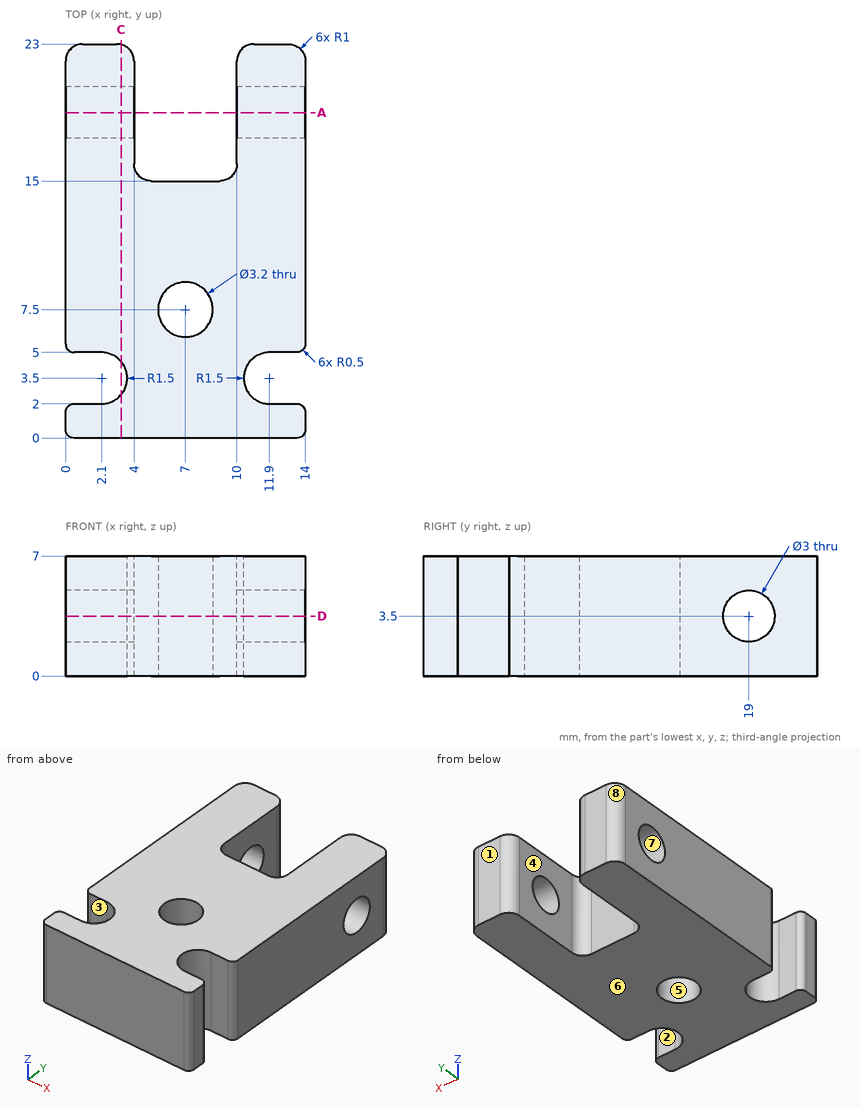
For this review, use the dimensioned drawing (mm, ordinates from the lowest corner) and the shaded views. A direction names the side the tool comes from. Coordinates: 2 decimals unless noted, no trailing zeros. Loops run counter-clockwise (first coordinate to the right, second up) from the corner with the lowest first, then second, coordinate; pieces in that order, holes last. Notation, with made-up numbers: (82, 61.5) - (135, 61.5) arc R16 ccw to (135, 91.5) - close; hole circle Ø5 at (28, 23). An arc over 180 degrees is marked (long way). Use CSV: the item, a comma, the result in double quotes. Start each with the question number.
1) Consider section D-D on z = 3.5. Give the number of separate pieces and of enclosed holes in the cut face, then the cut area to 3 significant figures.
2) Consider section A-A on y = 19. Write out the cut boundary in (x, z).
3) Tool access review of the marked faces 1, 2, 3, 4 and 5: name each direction out of +Z, -Z, +X, -X, +Y, -Y from which nothing blocks a thin tool from reaching the whole face with its end or side.
4) Consider section C-C on x = 3.25. Write out the cut boundary in (y, z), then the cut area to 3 significant figures.
5) The part is to be moulded in two halves that separate along Z. For the marked faces 6, 7 and 8, say which applies: +Z half, -Z half, draft (parallel to the pull), parting line (faces both ways), or undercut.
6) For pin 1 Ø3 at (y, z) = (19, 3) entering from +X; pin 2 Ø1.5 at (x, z) = (4.5, 5) entering from +Y, all flat-tipped, find the tip position at first contact; note any pin that passes through.
7) Wall thickness on L1, parallel to Y at x = 1.1, z = 3.5; L2, parallel to Y at x = 12.5, z = 0.75; L3, parallel to Y at x = 7, z = 3.5: over which ranges is each line inside the solid? List them lowest first. Write a range as from..to.
Geometry says:
1,separate pieces,"3"
1,enclosed holes,"1"
1,area,"222 mm^2"
2,outline,"(0, 0) - (4, 0) - (4, 2) - (0, 2) - close; (0, 5) - (4, 5) - (4, 7) - (0, 7) - close; (10, 0) - (14, 0) - (14, 2) - (10, 2) - close; (10, 5) - (14, 5) - (14, 7) - (10, 7) - close"
3,face 1,"+Z, -Z, +X, -X, +Y"
3,face 2,"+Z, -Z, +X"
3,face 3,"+Z, -Z, -X"
3,face 4,"+Z, -Z, +Y"
3,face 5,"+Z, -Z"
4,outline,"(0, 0) - (2.54, 0) - (2.54, 7) - (0, 7) - close; (4.46, 0) - (22.97, 0) - (22.97, 7) - (4.46, 7) - close; hole circle Ø3 at (19, 3.5)"
4,area,"140 mm^2"
5,face 6,"-Z half"
5,face 7,"undercut"
5,face 8,"draft"
6,pin 1,"x = 14"
6,pin 2,"y = 22.66"
7,L1,"0..2, 5..17.5, 20.5..23"
7,L2,"0..2, 5..23"
7,L3,"0..5.9, 9.1..15"
